```python
from build123d import *
from OCP.BRepFilletAPI import BRepFilletAPI_MakeChamfer

# Parameters (mm, degrees)
BOSS_EXTRUDE1_DEPTH = 30
CUT_EXTRUDE1_REACH  = 253.063
SKETCH10_W          = 41.5
SKETCH10_H          = 34
BOSS_EXTRUDE3_DEPTH = 4
CHAMFER4_SIZE       = 20
CHAMFER4_SIZE2      = 11.547005384
SKETCH11_W          = 20.75
SKETCH11_H          = 166.64
BOSS_EXTRUDE4_DEPTH = 4
SKETCH12_W          = 20.75
SKETCH12_H          = 33.32
BOSS_EXTRUDE5_DEPTH = 4
SKETCH13_W          = 20
SKETCH13_H          = 60
SKETCH13_W_2        = 70
SKETCH13_H_2        = 20
CUT_EXTRUDE2_DEPTH  = 4
FILLET2_R           = 3
SKETCH14_R          = 1.6
CUT_EXTRUDE3_DEPTH  = 4
CUT_EXTRUDE4_START  = -2
SKETCH15_R          = 3.5
SKETCH15_R_2        = 1.6
CUT_EXTRUDE4_DEPTH  = 2


with BuildPart() as part:
    # Sketch6 → Boss-Extrude1 (new body)
    with BuildSketch(Plane(origin=(0, 0, 0), x_dir=(1, 0, 0), z_dir=(0, 1, 0))):
        Polygon((0, -87.32), (37.5, -87.32), (37.5, -117.32), (90.67, -117.32), (142.319755082, -87.5), (142.319755082, 87.5), (90.67, 117.32), (37.5, 117.32), (37.5, 87.32), (0, 87.32), (0, 83.32), (41.5, 83.32), (41.5, 113.32), (89.59820323, 113.32), (138.319755082, 85.190598923), (138.319755082, -85.190598923), (89.59820323, -113.32), (41.5, -113.32), (41.5, -83.32), (0, -83.32), align=None)
    extrude(amount=BOSS_EXTRUDE1_DEPTH)

    # Sketch9 → Cut-Extrude1 (cut, up to next)
    with BuildSketch(Plane.XY.offset(87.32), mode=Mode.PRIVATE) as cut_extrude1_sk1:
        Polygon((37.5, 0), (15, 8), (0, 8), (0, 0), align=None)
    cut_extrude1_tool1 = extrude(cut_extrude1_sk1.sketch, amount=-CUT_EXTRUDE1_REACH, mode=Mode.PRIVATE) & part.part
    cut_extrude1 = cut_extrude1_tool1.solids().sort_by_distance((13.928571, 3.428571, 87.32))[0]
    add(cut_extrude1, mode=Mode.SUBTRACT)

    # Sketch10 → Boss-Extrude3 (add)
    with BuildSketch(Plane(origin=(0, 30, 0), x_dir=(1, 0, 0), z_dir=(0, 1, 0))):
        with Locations((20.75, -100.32)):
            Rectangle(SKETCH10_W, SKETCH10_H)
    boss_extrude3 = extrude(amount=-BOSS_EXTRUDE3_DEPTH)

    # Mirror1: Cut-Extrude1, Boss-Extrude3 across plane
    add(cut_extrude1.mirror(Plane.XY), mode=Mode.SUBTRACT)
    add(boss_extrude3.mirror(Plane.XY))

    # Chamfer4: one chamfer whose edges measure the first distance from different faces: ONE call of the kernel's chamfer builder (chamfer() names one face for all edges)
    chamfer4_edges_1 = [part.edges().sort_by_distance(p)[0] for p in [
        (37.5, 26, -102.32),
    ]]
    chamfer4_side_1 = [part.faces().sort_by_distance(p)[0] for p in [
        (18.75, 26, -102.32),
    ]]
    chamfer4_edges_2 = [part.edges().sort_by_distance(p)[0] for p in [
        (37.5, 26, 102.32),
    ]]
    chamfer4_side_2 = [part.faces().sort_by_distance(p)[0] for p in [
        (18.75, 26, 102.32),
    ]]
    chamfer4 = BRepFilletAPI_MakeChamfer(part.part.solid().wrapped)
    for e in chamfer4_edges_1:
        chamfer4.Add(CHAMFER4_SIZE, CHAMFER4_SIZE2, e.wrapped, chamfer4_side_1[0].wrapped)  # the first distance lies on this face
    for e in chamfer4_edges_2:
        chamfer4.Add(CHAMFER4_SIZE, CHAMFER4_SIZE2, e.wrapped, chamfer4_side_2[0].wrapped)  # the first distance lies on this face
    add(Compound.cast(chamfer4.Shape()), mode=Mode.REPLACE)

    # Sketch11 → Boss-Extrude4 (add)
    with BuildSketch(Plane(origin=(0, 30, 0), x_dir=(1, 0, 0), z_dir=(0, 1, 0))):
        with Locations((10.375, 0)):
            Rectangle(SKETCH11_W, SKETCH11_H)
    extrude(amount=-BOSS_EXTRUDE4_DEPTH)

    # Sketch12 → Boss-Extrude5 (add)
    with BuildSketch(Plane(origin=(0, 30, 0), x_dir=(1, 0, 0), z_dir=(0, 1, 0))):
        Polygon((41.5, 50), (20.75, 50), (20.75, -50), (41.5, -50), (138.319755082, -50), (138.319755082, 50), align=None)
        with Locations((31.125, -66.66)):
            Rectangle(SKETCH12_W, SKETCH12_H)
        with Locations((31.125, 66.66)):
            Rectangle(SKETCH12_W, SKETCH12_H)
    extrude(amount=-BOSS_EXTRUDE5_DEPTH)

    # Sketch13 → Cut-Extrude2 (cut)
    with BuildSketch(Plane(origin=(0, 30, 0), x_dir=(1, 0, 0), z_dir=(0, 1, 0))):
        with Locations((24.909877541, 0)):
            Rectangle(SKETCH13_W, SKETCH13_H)
        with Locations((89.909877541, 20)):
            Rectangle(SKETCH13_W_2, SKETCH13_H_2)
        with Locations((89.909877541, -20)):
            Rectangle(SKETCH13_W_2, SKETCH13_H_2)
    extrude(amount=-CUT_EXTRUDE2_DEPTH, mode=Mode.SUBTRACT)

    # Fillet2
    fillet2_edges = [part.edges().sort_by_distance(p)[0] for p in [
        (54.909877541, 28, 30),
        (54.909877541, 28, 10),
        (124.909877541, 28, 10),
        (124.909877541, 28, 30),
        (34.909877541, 28, -30),
        (34.909877541, 28, 30),
        (14.909877541, 28, 30),
        (14.909877541, 28, -30),
        (54.909877541, 28, -10),
        (54.909877541, 28, -30),
        (124.909877541, 28, -30),
        (124.909877541, 28, -10),
    ]]
    fillet(fillet2_edges, radius=FILLET2_R)

    # Sketch14 → Cut-Extrude3 (cut)
    with BuildSketch(Plane(origin=(0, 30, 0), x_dir=(1, 0, 0), z_dir=(0, 1, 0))):
        with Locations(Location((39.997609887, -40.001015731, 0), (0, 0, 270))):
            Circle(SKETCH14_R)
        with Locations(Location((97.997609783, -40.004481411, 0), (0, 0, 270))):
            Circle(SKETCH14_R)
        with Locations(Location((40.002748653, 45.998984115, 0), (0, 0, 270))):
            Circle(SKETCH14_R)
        with Locations(Location((98.00274855, 45.995518435, 0), (0, 0, 270))):
            Circle(SKETCH14_R)
    extrude(amount=-CUT_EXTRUDE3_DEPTH, mode=Mode.SUBTRACT)

    # Sketch15 → Cut-Extrude4 (cut)
    # profile 1 of 8: a face of its own
    with BuildSketch(Plane.XZ.offset(-26).offset(CUT_EXTRUDE4_START)):
        with Locations(Location((40.002748653, -45.998984115, 0), (0, 0, 270))):
            Circle(SKETCH15_R)
        with Locations(Location((40.002748653, -45.998984115, 0), (0, 0, 90))):
            Circle(SKETCH15_R_2, mode=Mode.SUBTRACT)
    # profile 2 of 8: a face of its own
    with BuildSketch(Plane.XZ.offset(-26).offset(CUT_EXTRUDE4_START)):
        with BuildLine():
            Line((101.50274855, -50), (101.50274855, -45.995518435))
            ThreePointArc((101.50274855, -45.995518435), (98.00274855, -49.495518435), (94.50274855, -45.995518435))
            Line((94.50274855, -45.995518435), (94.50274855, -50))
            Line((94.50274855, -50), (101.50274855, -50))
        make_face()
    # profile 3 of 8: a face of its own
    with BuildSketch(Plane.XZ.offset(-26).offset(CUT_EXTRUDE4_START)):
        with BuildLine():
            ThreePointArc((94.50274855, -45.995518435), (98.00274855, -49.495518435), (101.50274855, -45.995518435))
            Line((101.50274855, -45.995518435), (99.60274855, -45.995518435))
            ThreePointArc((99.60274855, -45.995518435), (98.00274855, -47.595518435), (96.40274855, -45.995518435))
            Line((96.40274855, -45.995518435), (94.50274855, -45.995518435))
        make_face()
    # profile 4 of 8: a face of its own
    with BuildSketch(Plane.XZ.offset(-26).offset(CUT_EXTRUDE4_START)):
        with BuildLine():
            Line((99.60274855, -45.995518435), (101.50274855, -45.995518435))
            ThreePointArc((101.50274855, -45.995518435), (98.00274855, -42.495518435), (94.50274855, -45.995518435))
            Line((94.50274855, -45.995518435), (96.40274855, -45.995518435))
            ThreePointArc((96.40274855, -45.995518435), (98.00274855, -44.395518435), (99.60274855, -45.995518435))
        make_face()
    # profile 5 of 8: a face of its own
    with BuildSketch(Plane.XZ.offset(-26).offset(CUT_EXTRUDE4_START)):
        with BuildLine():
            ThreePointArc((94.50274855, -45.995518435), (98.00274855, -49.495518435), (101.50274855, -45.995518435))
            Line((101.50274855, -45.995518435), (99.60274855, -45.995518435))
            ThreePointArc((99.60274855, -45.995518435), (98.00274855, -47.595518435), (96.40274855, -45.995518435))
            Line((96.40274855, -45.995518435), (94.50274855, -45.995518435))
        make_face()
    # profile 6 of 8: a face of its own
    with BuildSketch(Plane.XZ.offset(-26).offset(CUT_EXTRUDE4_START)):
        with BuildLine():
            Line((99.60274855, -45.995518435), (101.50274855, -45.995518435))
            ThreePointArc((101.50274855, -45.995518435), (98.00274855, -42.495518435), (94.50274855, -45.995518435))
            Line((94.50274855, -45.995518435), (96.40274855, -45.995518435))
            ThreePointArc((96.40274855, -45.995518435), (98.00274855, -44.395518435), (99.60274855, -45.995518435))
        make_face()
    # profile 7 of 8: a face of its own
    with BuildSketch(Plane.XZ.offset(-26).offset(CUT_EXTRUDE4_START)):
        with Locations(Location((97.997609783, 40.004481411, 0), (0, 0, 270))):
            Circle(SKETCH15_R)
        with Locations(Location((97.997609783, 40.004481411, 0), (0, 0, 90))):
            Circle(SKETCH15_R_2, mode=Mode.SUBTRACT)
    # profile 8 of 8: a face of its own
    with BuildSketch(Plane.XZ.offset(-26).offset(CUT_EXTRUDE4_START)):
        with Locations(Location((39.997609887, 40.001015731, 0), (0, 0, 270))):
            Circle(SKETCH15_R)
        with Locations(Location((39.997609887, 40.001015731, 0), (0, 0, 90))):
            Circle(SKETCH15_R_2, mode=Mode.SUBTRACT)
    extrude(amount=CUT_EXTRUDE4_DEPTH, mode=Mode.SUBTRACT)


solid = part.part
```
Can you work these out from the model? Positions are in its coordinate system, mm. A direction names the side the tool comes from. Round coordinates to 2 decimals unless told otherwise and drop trailing zeros. Loops run counter-clockwise (first coordinate to the right, second up) from the corner with the lowest first, then second, coordinate; pieces in that order, holes last. Notation, with made-up numbers: M -35.75,-24.5 L -1.75,-24.5 A15 cw -1.75,-10.5 Z; hole C -2.75,-6 d9. An arc over 180 degrees is marked long. Answer as a JSON object with one key per item and string values. Group by question number.
Q1. We'd pull the mould along X, two halves only. Please class faces 4 (the flat face through (66, 15, 113.32)), 5 (the flat face through (114.3, 14.79, 99.06)), 6 (the flat face through (55, 15, 117.32)), 7 (the flat face through (26.408, 3.944, 85.348)): +X half, -X half, draft (parallel to the pull), parting line (faces both ways), or undercut.
Q2. Please list where these lines run through material, in increasing order: L1, parallel to Z at x = 32, y = 26.75; L2, parallel to Z at x = 15, y = 19.5; L3, parallel to X at y = 26.25, z = 74.5.
Q3. On a 3-axis mill with a long thin cutter (end or side, diameter ignored), from which of +Z, -Z, +X, -X, +Y, -Y can I reach the whole of each face in a straight line? I mean faces 1 (the flat face through (38, 28, 39)), 2 (the flat face through (65, 15, -113.32)), 3 (the flat face through (18, 16, 87.32)). Say none if no direction works.
Q4. Imagine slicing it at B-B, the plane x = 24. Please give me the cut outline in (y, z), then the cut area to 3 significant figures.
Q5. Imagine slicing it at C-C, the plane y = 10.25. Please give me the cut outline in (x, z), then the cut area to 3 significant figures.
Q6. Imagine slicing it at D-D, the plane x = 117. Please give me the cut outline in (y, z), then the cut area to 3 significant figures.
Q7. Will these pins go through, and if not, where does the flat tip stop? pin 1 (7.5 mm diameter, centred on x = 41, z = 41.5, fed in from -Y); pin 2 (3 mm diameter, centred on y = 7.5, z = -63, fed in from -X); pin 3 (1.2 mm diameter, centred on x = 114, y = 28.5, fed in from -Z); pin 4 (3 mm diameter, centred on x = 98, z = -46, fed in from -Y).
Q8. Imagine slicing it at A-A, the plane z = 75. Please give me the cut outline in (x, y), then the cut area to 3 significant figures.
Findings:
{
 "1": {"face 4": "undercut", "face 5": "undercut", "face 6": "draft", "face 7": "-X half"},
 "2": {"L1": "z = -117.32 to -30, 30 to 117.32", "L2": "z = -87.32 to -83.32, 83.32 to 87.32", "L3": "x = 0 to 41.5, 138.32 to 142.32"},
 "3": {"face 1": "-Y", "face 2": "+Y, -Y", "face 3": "+Z, -X, -Y"},
 "4": {"outline": "M 4.8,-87.32 L 22.25,-87.32 L 22.25,-117.32 L 30,-117.32 L 30,-30 L 26,-30 L 26,-83.32 L 4.8,-83.32 Z; M 4.8,83.32 L 26,83.32 L 26,30 L 30,30 L 30,117.32 L 22.25,117.32 L 22.25,87.32 L 4.8,87.32 Z", "area": "1,090 mm2"},
 "5": {"outline": "M 0,-87.32 L 37.5,-87.32 L 37.5,-117.32 L 90.67,-117.32 L 142.32,-87.5 L 142.32,87.5 L 90.67,117.32 L 37.5,117.32 L 37.5,87.32 L 0,87.32 L 0,83.32 L 41.5,83.32 L 41.5,113.32 L 89.6,113.32 L 138.32,85.19 L 138.32,-85.19 L 89.6,-113.32 L 41.5,-113.32 L 41.5,-83.32 L 0,-83.32 Z", "area": "2,120 mm2"},
 "6": {"outline": "M 0,-102.12 L 30,-102.12 L 30,-97.5 L 0,-97.5 Z; M 0,97.5 L 30,97.5 L 30,102.12 L 0,102.12 Z; M 26,-50 L 30,-50 L 30,-30 L 26,-30 Z; M 26,-10 L 30,-10 L 30,10 L 26,10 Z; M 26,30 L 30,30 L 30,50 L 26,50 Z", "area": "517 mm2"},
 "7": {"pin 1": "stops at y = 26", "pin 2": "stops at x = 138.32", "pin 3": "stops at z = -104.2", "pin 4": "passes through"},
 "8": {"outline": "M 0,26 L 41.5,26 L 41.5,30 L 0,30 Z; M 138.32,0 L 142.32,0 L 142.32,30 L 138.32,30 Z", "area": "286 mm2"}
}
